Can you work these out from the model? Positions are in its coordinate system, mm. Face numbers are marked on the shaded views. Coordinates: 2 decimals unless noted, no trailing zeros. Loops run counter-clockwise (first coordinate to the right, second up) from the corner with the lowest first, then second, coordinate; pieces in that order, holes last.
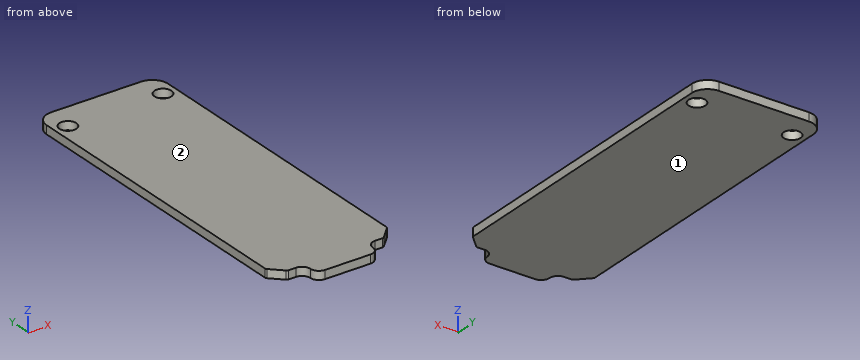
```python
from build123d import *

# Parameters (mm, degrees)
BOSS_EXTRUDE1_DEPTH  = 1.6
FILLET1_R            = 3
FILLET2_START        = -1
FILLET2_DEPTH        = 4
FILLET2_2_DEPTH      = 1.6
FILLET3_R            = 0.5
M3_CLEARANCE_HOLE1_D = 3.2


with BuildPart() as part:
    # Sketch1 → Boss-Extrude1 (new body)
    with BuildSketch(Plane.XY):
        Polygon((11.5, 83.1), (-11.5, 83.1), (-11.5, 22.6), (-9.1, 20.2), (-5.9, 20.2), (-5.9, 17), (5.9, 17), (5.9, 20.2), (9.1, 20.2), (11.5, 22.6), align=None)
    extrude(amount=BOSS_EXTRUDE1_DEPTH)

    # Fillet1
    fillet1_edges = [part.edges().sort_by_distance(p)[0] for p in [
        (-11.5, 83.1, 0.8),
        (11.5, 83.1, 0.8),
    ]]
    fillet(fillet1_edges, radius=FILLET1_R)

    # Fillet2: read off the stored shape, not the designer's step
    # Fillet2 outline → Fillet2 (cut)
    with BuildSketch(Plane.XY.offset(FILLET2_START)):
        with BuildLine():
            ThreePointArc((5.9, 18.6), (5.43137085, 17.46862915), (4.3, 17))
            Line((4.3, 17), (5.9, 17))
            Line((5.9, 17), (5.9, 18.6))
        make_face()
        with BuildLine():
            ThreePointArc((-4.3, 17), (-5.43137085, 17.46862915), (-5.9, 18.6))
            Line((-5.9, 18.6), (-5.9, 17))
            Line((-5.9, 17), (-4.3, 17))
        make_face()
    extrude(amount=FILLET2_DEPTH, mode=Mode.SUBTRACT)

    # Fillet2 2 outline → Fillet2 2 (add)
    with BuildSketch(Plane.XY):
        with BuildLine():
            Line((5.9, 20.2), (5.9, 18.6))
            ThreePointArc((5.9, 18.6), (6.36862915, 19.73137085), (7.5, 20.2))
            Line((7.5, 20.2), (5.9, 20.2))
        make_face()
        with BuildLine():
            ThreePointArc((-7.5, 20.2), (-6.36862915, 19.73137085), (-5.9, 18.6))
            Line((-5.9, 18.6), (-5.9, 20.2))
            Line((-5.9, 20.2), (-7.5, 20.2))
        make_face()
    extrude(amount=FILLET2_2_DEPTH)

    # Fillet3
    fillet3_edges = [part.edges().sort_by_distance(p)[0] for p in [
        (-11.5, 22.6, 0.8),
        (11.5, 22.6, 0.8),
        (9.1, 20.2, 0.8),
        (-9.1, 20.2, 0.8),
    ]]
    fillet(fillet3_edges, radius=FILLET3_R)

    # M3 Clearance Hole1 (through all)
    with Locations(Plane.XY.offset(1.6)):
        with Locations((-9, 78), (9, 78)):
            Hole(M3_CLEARANCE_HOLE1_D / 2)


solid = part.part
```
(1) If we mould it in two halves opening along Z, with no side actions, what happens to the marked faces 1 and 2? For each: released by +Z, released by -Z, zero draft, split by the parting line, or undercut.
Check values:
face 1: released by -Z
face 2: released by +Z
(2) I want a section at A-A on z = 1. Write out the boundary of the cut face in (x, y), then the cut area to 3 significant figures.
Check values:
outline: (-11.5, 22.81) arc R0.5 ccw to (-11.35, 22.45) - (-9.25, 20.35) arc R0.5 ccw to (-8.89, 20.2) - (-7.5, 20.2) arc R1.6 cw to (-5.9, 18.6) arc R1.6 ccw to (-4.3, 17) - (4.3, 17) arc R1.6 ccw to (5.9, 18.6) arc R1.6 cw to (7.5, 20.2) - (8.89, 20.2) arc R0.5 ccw to (9.25, 20.35) - (11.35, 22.45) arc R0.5 ccw to (11.5, 22.81) - (11.5, 80.1) arc R3 ccw to (8.5, 83.1) - (-8.5, 83.1) arc R3 ccw to (-11.5, 80.1) - close; hole circle Ø3.2 at (-9, 78); hole circle Ø3.2 at (9, 78)
area: 1,460 mm2
(3) If I drill on probe 1 along X at (y, z) = (78, 0.55); probe 2 along Y at (x, z) = (-9, 0.6); probe 3 along Y at (x, z) = (-7.25, 1.45), over which ranges is the centre line in solid material (lowest first)?
Check values:
probe 1: x = -11.5 to -10.6, -7.4 to 7.4, 10.6 to 11.5
probe 2: y = 20.21 to 76.4, 79.6 to 83.06
probe 3: y = 20.18 to 83.1
